from build123d import *

# Parameters (mm, degrees)
F0_W     = 164
F0_H     = 170
F0_R     = 6
F0_R_2   = 7
F1_DEPTH = 5
F2_W     = 20
F2_H     = 5
F3_DEPTH = 0.01


with BuildPart() as f1:
    # F0 (on Top) → F1 (new body)
    with BuildSketch(Plane.XY):
        Rectangle(F0_W, F0_H)
        with Locations((-66.75, 0)):
            Circle(F0_R, mode=Mode.SUBTRACT)
        with Locations((0, 40)):
            Circle(F0_R_2, mode=Mode.SUBTRACT)
        with Locations((66.75, 0)):
            Circle(F0_R, mode=Mode.SUBTRACT)
    extrude(amount=F1_DEPTH)

    # F2 (on face) → F3 (join)
    with BuildSketch(Plane(origin=(0, 85, 0), x_dir=(-1, 0, 0), z_dir=(0, 1, 0))):
        with Locations((72, 2.5)):
            Rectangle(F2_W, F2_H)
        with Locations((-72, 2.5)):
            Rectangle(F2_W, F2_H)
    extrude(amount=-F3_DEPTH)


solid = f1.part
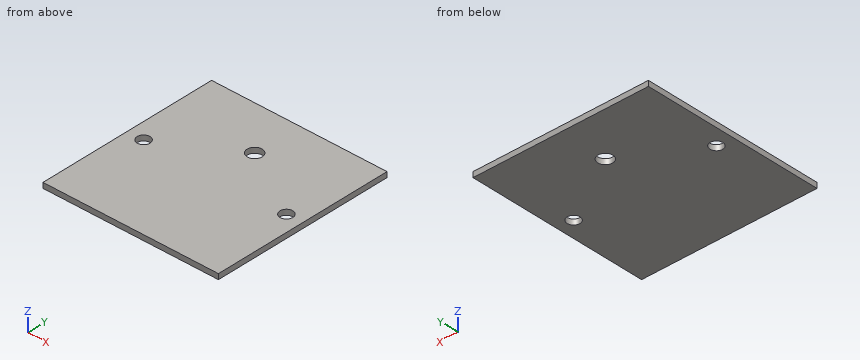
Can you work these out from the model? Positions are in its coordinate system, mm. Coordinates: 2 decimals unless noted, no trailing zeros. Order: outer loops, then holes, each group sorted by start corner. A loop starts at its lowest first (then second) coordinate and runs counter-clockwise, first axis right, second up. Notation, with made-up numbers: (58.25, 83.5) - (113.25, 83.5) arc R25 ccw to (113.25, 113.5) - close; hole circle Ø4 at (39.5, 49). An arc over 180 degrees is marked (long way). Answer as a JSON object with one key per item and string values. Group by question number.
Q1. Imagine slicing it at B-B (x = -66.75). Please give me the cut outline in (y, z).
Q2. Imagine slicing it at C-C (y = 40). Please give me the cut outline in (x, z), and give its area (3 significant figures).
Q3. Imagine slicing it at A-A (y = 0). Please give me the cut outline in (x, z), and give its area (3 significant figures).
Q4. I need wall thicknesses on line 1 (Y direction, x = 0, z = 2.35); line 2 (Y direction, x = 66.75, z = 2.45); line 3 (X direction, y = 1, z = 3.1). Which ranges of each line are inside material? Lowest first, please. Write a range as from..to.
Q5. Will these pins go through, and if not, where does the flat tip stop? P1, Ø7, axis at x = -66.75, y = 0, coming from the -Z side; P2, Ø10, axis at x = 63, y = -22.5, coming from the -Z side.
Determined:
{
 "1": {"outline": "(-85, 0) - (-6, 0) - (-6, 5) - (-85, 5) - close; (6, 0) - (85, 0) - (85, 5) - (6, 5) - close"},
 "2": {"outline": "(-82, 0) - (-7, 0) - (-7, 5) - (-82, 5) - close; (7, 0) - (82, 0) - (82, 5) - (7, 5) - close", "area": "750 mm2"},
 "3": {"outline": "(-82, 0) - (-72.75, 0) - (-72.75, 5) - (-82, 5) - close; (-60.75, 0) - (60.75, 0) - (60.75, 5) - (-60.75, 5) - close; (72.75, 0) - (82, 0) - (82, 5) - (72.75, 5) - close", "area": "700 mm2"},
 "4": {"line 1": "y = -85..33, 47..85", "line 2": "y = -85..-6, 6..85", "line 3": "x = -82..-72.67, -60.83..60.83, 72.67..82"},
 "5": {"P1": "passes through", "P2": "stops at z = 0"}
}
